Verification items for this drawing (mm, ordinates from the low corner). A direction names the side the tool comes from. Give positions to 0.01 mm unless a question says otherwise; leave off trailing zeros. Loops run counter-clockwise (first coordinate to the right, second up) from the corner with the lowest first, then second, coordinate; pieces in that order, holes last. Notation, with made-up numbers: M 2,32 L 59,32 A11 ccw 59,47 Z; hole C 73,-3.5 d2. An arc over 180 degrees is marked long. Use one line per item in the form item = value.
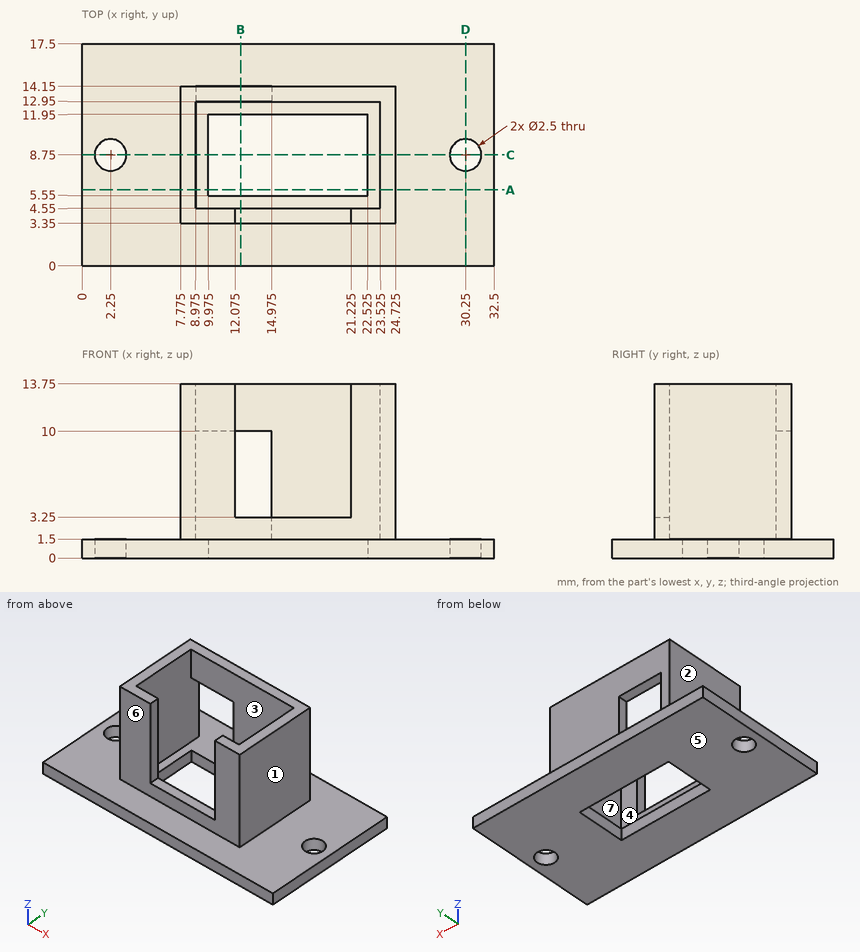
1) Scan lines: line 1 (Y direction, x = 30.25, z = 0.55); line 2 (Y direction, x = 19.5, z = 2); line 3 (Z direction, x = 10, y = 13.75). Record each from-to range of solid material in increasing order.
Evaluation:
line_1 = 0 to 7.5, 10 to 17.5
line_2 = 3.35 to 4.55, 12.95 to 14.15
line_3 = 0 to 1.5, 10 to 13.75
2) Release check for a two-part mould opening along Y. For the marked faces 4, 5, 6 and 7 record: pulls with the +Y half, pulls with the -Y half, needs draft (parallel to the pull), parting line crosses it, or undercut.
Evaluation:
face_4 = undercut
face_5 = needs draft
face_6 = pulls with the -Y half
face_7 = undercut
3) Section check A-A (y = 6). Record the cut outline in (x, z) (3 decimals), then the cut area to 3 significant figures.
Evaluation:
outline = M 0,0 L 9.975,0 L 9.975,1.5 L 8.975,1.5 L 8.975,13.75 L 7.775,13.75 L 7.775,1.5 L 0,1.5 Z; M 22.525,0 L 32.5,0 L 32.5,1.5 L 24.725,1.5 L 24.725,13.75 L 23.525,13.75 L 23.525,1.5 L 22.525,1.5 Z
area = 59.3 mm^2
4) Section check C-C (y = 8.75). Record the cut outline in (x, z) (3 decimals), then the cut area to 3 significant figures.
Evaluation:
outline = M 0,0 L 1,0 L 1,1.5 L 0,1.5 Z; M 3.5,0 L 9.975,0 L 9.975,1.5 L 8.975,1.5 L 8.975,13.75 L 7.775,13.75 L 7.775,1.5 L 3.5,1.5 Z; M 22.525,0 L 29,0 L 29,1.5 L 24.725,1.5 L 24.725,13.75 L 23.525,13.75 L 23.525,1.5 L 22.525,1.5 Z; M 31.5,0 L 32.5,0 L 32.5,1.5 L 31.5,1.5 Z
area = 51.8 mm^2
5) Set-up check for the marked faces 1, 2 and 3: record each of +Z, -Z, +X, -X, +Y, -Y from which the full face is reachable in a straight line by a thin tool's end or side.
Evaluation:
face_1 = +Z, +X, +Y, -Y
face_2 = +Z, -X, +Y, -Y
face_3 = +Z
6) Depth check by flat-ended pin: pin 1 Ø4 at (x, y) = (10.5, 10.5) entering from -Z; pin 2 Ø1 at (x, y) = (16, 4) entering from +Z; pin 3 Ø1 at (y, z) = (3.5, 9) entering from -X (3 decimals); pin 4 Ø6 at (x, z) = (19, 6) entering from -Y. Enter the tip coordinate at first touch or a pass-through.
Evaluation:
pin_1 = 0
pin_2 = 3.25
pin_3 = 7.775
pin_4 = 3.35
7) Section check D-D (x = 30.25). Record the cut outline in (y, z), then the cut area to 3 significant figures.
Evaluation:
outline = M 0,0 L 7.5,0 L 7.5,1.5 L 0,1.5 Z; M 10,0 L 17.5,0 L 17.5,1.5 L 10,1.5 Z
area = 22.5 mm^2
8) Section check B-B (x = 12.5). Record the cut outline in (y, z).
Evaluation:
outline = M 0,0 L 5.55,0 L 5.55,1.5 L 4.55,1.5 L 4.55,3.25 L 3.35,3.25 L 3.35,1.5 L 0,1.5 Z; M 11.95,0 L 17.5,0 L 17.5,1.5 L 11.95,1.5 Z; M 12.95,10 L 14.15,10 L 14.15,13.75 L 12.95,13.75 Z
